Geometry check sheet. Reference: drawing and pictorial views, mm from the part's lowest x, y, z. A direction names the side the tool comes from. Round coordinates to 2 decimals unless told otherwise and drop trailing zeros. Write each loop counter-clockwise with the first axis right and the second up, starting at its lowest first coordinate (ties: lowest second). Pieces come first, ordered by that corner, then holes. Notation, with made-up numbers: M -19.5,45 L 4.5,45 A14 cw 4.5,54 Z; hole C -37.75,49.5 d4. An arc over 180 degrees is marked long. Answer in a Markdown table with one row per item.
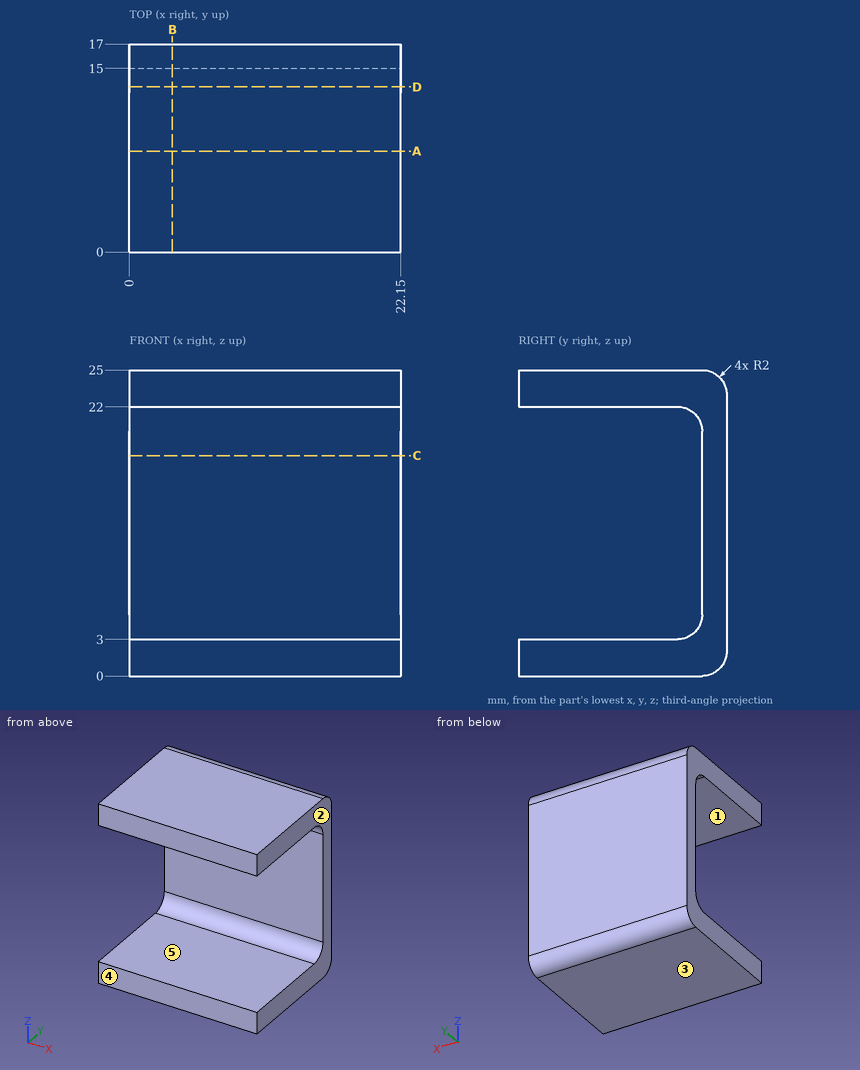
1. Section check D-D, the plane y = 13.5. Record the cut outline in (x, z), and give its area (3 significant figures).
Found:
| item | result |
|---|---|
| outline | M 0,0 L 22.15,0 L 22.15,3.06 L 0,3.06 Z; M 0,21.94 L 22.15,21.94 L 22.15,25 L 0,25 Z |
| area | 136 mm2 |
2. Draft check along Z on the marked faces 1, 2 and 3. Enter one of: +Z half, -Z half, draft (parallel to the pull), parting line (faces both ways), or undercut.
Found:
| item | result |
|---|---|
| face 1 | undercut |
| face 2 | draft |
| face 3 | -Z half |
3. Section check A-A, the plane y = 8.25. Record the cut outline in (x, z), and give its area (3 significant figures).
Found:
| item | result |
|---|---|
| outline | M 0,0 L 22.15,0 L 22.15,3 L 0,3 Z; M 0,22 L 22.15,22 L 22.15,25 L 0,25 Z |
| area | 133 mm2 |
4. Access from +Z, -Z, +X, -X, +Y, -Y to the whole of each face (thin tool, end or side, straight path). Record for the marked faces 4 and 5.
Found:
| item | result |
|---|---|
| face 4 | +Z, -Z, +X, -X, -Y |
| face 5 | +X, -X, -Y |
5. Section check C-C, the plane z = 18. Record the cut outline in (x, y), and give its area (3 significant figures).
Found:
| item | result |
|---|---|
| outline | M 0,15 L 22.15,15 L 22.15,17 L 0,17 Z |
| area | 44.3 mm2 |
6. Section check B-B, the plane x = 3.5. Record the cut outline in (y, z), and give its area (3 significant figures).
Found:
| item | result |
|---|---|
| outline | M 0,0 L 15,0 A2 ccw 17,2 L 17,23 A2 ccw 15,25 L 0,25 L 0,22 L 13,22 A2 cw 15,20 L 15,5 A2 cw 13,3 L 0,3 Z |
| area | 140 mm2 |
7. Go/stop test with a flat-tipped pin: pin 1 (4 mm diameter, centred on x = 3, z = 14.5, fed in from -Y). Record where the tip stops, or that it passes through.
Found:
| item | result |
|---|---|
| pin 1 | stops at y = 15 |
8. Scan lines: L1, parallel to Z at x = 7.5, y = 10.5; L2, parallel to Y at x = 17, z = 15; L3, parallel to Z at x = 11.5, y = 13.75. Record each from-to range of solid material in increasing order.
Found:
| item | result |
|---|---|
| L1 | z = 0 to 3, 22 to 25 |
| L2 | y = 15 to 17 |
| L3 | z = 0 to 3.15, 21.85 to 25 |
